from build123d import *

# Parameters (mm, degrees)
F0_R     = 46.99
F0_R_2   = 3.175
F1_DEPTH = 1.27


with BuildPart() as f1:
    # F0 (on Top) → F1 (new body)
    with BuildSketch(Plane.XY):
        Circle(F0_R)
        with Locations((0, -23.20925)):
            Circle(F0_R_2, mode=Mode.SUBTRACT)
        with Locations((-11.1125, -11.1125)):
            Circle(F0_R_2, mode=Mode.SUBTRACT)
        with Locations((11.1125, -11.1125)):
            Circle(F0_R_2, mode=Mode.SUBTRACT)
        with BuildLine():
            ThreePointArc((1.5875, 9.211406), (7.148735, 6.022104), (9.3472, 0))
            ThreePointArc((9.3472, 0), (-6.022104, -7.148735), (-1.5875, 9.211406))
            Line((-1.5875, 9.211406), (-1.5875, 10.033))
            Line((-1.5875, 10.033), (1.5875, 10.033))
            Line((1.5875, 10.033), (1.5875, 9.211406))
        make_face(mode=Mode.SUBTRACT)
        with Locations((-11.1125, 11.1125)):
            Circle(F0_R_2, mode=Mode.SUBTRACT)
        with Locations((11.1125, 11.1125)):
            Circle(F0_R_2, mode=Mode.SUBTRACT)
    extrude(amount=F1_DEPTH)


solid = f1.part
Design review of the part built by this model. Coordinates are the model's own, in mm. Round coordinates to 2 decimals unless told otherwise and drop trailing zeros. Write each loop counter-clockwise with the first axis right and the second up, starting at its lowest first coordinate (ties: lowest second). Pieces come first, ordered by that corner, then holes. Notation, with made-up numbers: (-10.5, 20.25) - (12.5, 20.25) arc R20 ccw to (12.5, 50.25) - close; hole circle Ø3 at (68.25, 74). An arc over 180 degrees is marked (long way). Return JSON: item names as keys, results as strings. Group by question number.
Item 1: The part is to be moulded in two halves that separate along Y. For faces 1 (the face through (10, 1, 1.27)), 2 (the face through (-10.19, -45.87, 0.63)), 3 (the face through (10.699, -7.965, 0.626)), say which applies: pulls with the +Y half, pulls with the -Y half, needs draft (parallel to the pull), parting line crosses it, or undercut.
Item 2: For probe 1 along Y at (x, z) = (0, 0.7); probe 2 along X at (y, z) = (-14, 0.95); probe 3 along X at (y, z) = (-22, 0.85), list the stretches that pass through material, from the lowest coordinate up. Write a range as [from, to].
Item 3: We need section B-B on z = 0.8. Give the number of separate pieces and of enclosed holes in the cut face, and give its area (3 significant figures).
Item 4: We need section C-C on y = 36.5. Write out the cut boundary in (x, z).
Item 5: We need section A-A on x = 0. Write out the cut boundary in (y, z).
Item 6: We need section D-D on x = 20.5. Write out the cut boundary in (y, z), and give its area (3 significant figures).
Model answer:
{
 "1": {"face 1": "needs draft", "face 2": "parting line crosses it", "face 3": "undercut"},
 "2": {"probe 1": "y = [-46.99, -26.38], [-20.03, -9.35], [10.03, 46.99]", "probe 2": "x = [-44.86, -12.43], [-9.79, 9.79], [12.43, 44.86]", "probe 3": "x = [-41.52, -2.94], [2.94, 41.52]"},
 "3": {"separate pieces": "1", "enclosed holes": "6", "area": "6,500 mm²"},
 "4": {"outline": "(-29.59, 0) - (29.59, 0) - (29.59, 1.27) - (-29.59, 1.27) - close"},
 "5": {"outline": "(-46.99, 0) - (-26.38, 0) - (-26.38, 1.27) - (-46.99, 1.27) - close; (-20.03, 0) - (-9.35, 0) - (-9.35, 1.27) - (-20.03, 1.27) - close; (10.03, 0) - (46.99, 0) - (46.99, 1.27) - (10.03, 1.27) - close"},
 "6": {"outline": "(-42.28, 0) - (42.28, 0) - (42.28, 1.27) - (-42.28, 1.27) - close", "area": "107 mm²"}
}
